For this review, take the finished solid that the model builds, in its own axes (mm). Round coordinates to 2 decimals unless told otherwise and drop trailing zeros. Loops run counter-clockwise (first coordinate to the right, second up) from the corner with the lowest first, then second, coordinate; pieces in that order, holes last.
1. To check wall thickness, follow line 1 along X through (y, z) = (2, 0.2); line 2 along X through (y, z) = (9.25, 0.25); line 3 along Z through (x, y) = (28.5, 16.5) (1 decimal). State the ranges of each line that lie inside material, in increasing order.
2. Consider section A-A on x = 23. State the section outline as (y, z) points, then the cut area to 3 significant figures.
3. Consider section B-B on y = 9. State the section outline as (x, z) points, then the cut area to 3 significant figures.
4. Draft analysis for pull direction X (two halves, no side actions). For faces 1 (the flat face through (14.79, 1.01, 0.19)), 2 (the flat face through (31.6, 2.8, 0.4)), 3 (the cylindrical face through (21, 7.5, 0.4)), state which applies: released by +X, released by -X, zero draft, split by the parting line, or undercut.
5. Consider section C-C on z = 0.6. State the section outline as (x, y) points, then the cut area to 3 significant figures.
6. Consider section D-D on x = 10. State the section outline as (y, z) points.
from build123d import *

# Parameters (mm, degrees)
PAD_DEPTH       = 0.75
SKETCH001_R     = 2.5
POCKET_DEPTH    = 0.751
POCKET001_DEPTH = 35.001


with BuildPart() as part:
    # Sketch (on XY_Plane of Origin) → Pad (new body)
    with BuildSketch(Plane.XY):
        Polygon((0, 0), (0, 18), (26, 18), (35, 13.5), (35, 4.5), (26, 0), align=None)
    extrude(amount=PAD_DEPTH)

    # Sketch001 (on Face8 of Pad) → Pocket (cut, through all)
    with BuildSketch(Plane.XY.offset(0.75)):
        with Locations((23, 9)):
            Circle(SKETCH001_R)
    extrude(amount=-POCKET_DEPTH, mode=Mode.SUBTRACT)

    # Sketch002 (on Face1 of Pocket) → Pocket001 (cut, through all)
    with BuildSketch(Plane(origin=(0, 0, 0), x_dir=(0, -1, 0), z_dir=(-1, 0, 0))):
        Polygon((-2, 0), (0, 0.38), (-2, 0.75), (0, 0.75), (0, 0), align=None)
        Polygon((-16, 0.75), (-18, 0.38), (-16, 0), (-18, 0), (-18, 0.75), align=None)
    extrude(amount=-POCKET001_DEPTH, mode=Mode.SUBTRACT)


solid = part.part
Resolved:
1. line 1: x = 0 to 30
1. line 2: x = 0 to 20.51, 25.49 to 35
1. line 3: z = 0.1 to 0.7
2. outline: (0, 0.38) - (2, 0) - (6.5, 0) - (6.5, 0.75) - (2, 0.75) - close; (11.5, 0) - (16, 0) - (18, 0.38) - (16, 0.75) - (11.5, 0.75) - close
2. area: 8.25 mm2
3. outline: (0, 0) - (20.5, 0) - (20.5, 0.75) - (0, 0.75) - close; (25.5, 0) - (35, 0) - (35, 0.75) - (25.5, 0.75) - close
3. area: 22.5 mm2
4. face 1: zero draft
4. face 2: released by +X
4. face 3: undercut
5. outline: (0, 1.19) - (28.38, 1.19) - (35, 4.5) - (35, 13.5) - (28.38, 16.81) - (0, 16.81) - close; hole circle Ø5 at (23, 9)
5. area: 505 mm2
6. outline: (0, 0.38) - (2, 0) - (16, 0) - (18, 0.38) - (16, 0.75) - (2, 0.75) - close
